from build123d import *

# Parameters (mm, degrees)
SKETCH1_R           = 3.175
BOSS_EXTRUDE1_DEPTH = 25.4
SKETCH2_W           = 6.268193042
SKETCH2_H           = 1.016
BOSS_EXTRUDE2_DEPTH = 6.35
SKETCH3_R           = 1.27
CUT_EXTRUDE1_DEPTH  = 33.120205697
FILLET1_R           = 0.508


with BuildPart() as part:
    # Sketch1 → Boss-Extrude1 (new body)
    with BuildSketch(Plane(origin=(0, 0, 0), x_dir=(0, 0, -1), z_dir=(1, 0, 0))):
        Circle(SKETCH1_R)
    extrude(amount=BOSS_EXTRUDE1_DEPTH)

    # Sketch2 → Boss-Extrude2 (add)
    with BuildSketch(Plane(origin=(25.4, 0, 0), x_dir=(0, 0, -1), z_dir=(1, 0, 0))):
        Rectangle(SKETCH2_W, SKETCH2_H)
    extrude(amount=BOSS_EXTRUDE2_DEPTH)

    # Sketch3 → Cut-Extrude1 (cut, through all)
    with BuildSketch(Plane(origin=(0, 0.508, 0), x_dir=(1, 0, 0), z_dir=(0, 1, 0))):
        with Locations(Location((28.575, 0, 0), (0, 0, 270))):
            Circle(SKETCH3_R)
    extrude(amount=-CUT_EXTRUDE1_DEPTH, mode=Mode.SUBTRACT)

    # Fillet1
    # the kernel refuses this fillet: 0.508 mm, written as the material it adds along each edge
    with BuildSketch(Plane(origin=(25.4, -0.508, -3.134096521), x_dir=(0, -1, 0), z_dir=(0, 0, 1))) as fillet1_piece_1_section:
        with BuildLine():
            CenterArc((FILLET1_R, FILLET1_R), FILLET1_R, 180, 90)
            Line((0, FILLET1_R), (0, 0))
            Line((0, 0), (FILLET1_R, 0))
        make_face()
    fillet1_piece_1 = extrude(amount=6.268193041, mode=Mode.PRIVATE)
    fillet1_piece_1 = fillet1_piece_1 & Plane(origin=(25.515488837, 0, 0), x_dir=(0, 0, -1), z_dir=(-1, 0, 0)) * Cylinder(3.175, 15, mode=Mode.PRIVATE)
    add(fillet1_piece_1)
    with BuildSketch(Plane(origin=(25.4, 0.508, 3.134096521), x_dir=(0, 1, 0), z_dir=(0, 0, -1))) as fillet1_piece_2_section:
        with BuildLine():
            CenterArc((FILLET1_R, FILLET1_R), FILLET1_R, 180, 90)
            Line((0, FILLET1_R), (0, 0))
            Line((0, 0), (FILLET1_R, 0))
        make_face()
    fillet1_piece_2 = extrude(amount=6.268193041, mode=Mode.PRIVATE)
    fillet1_piece_2 = fillet1_piece_2 & Plane(origin=(25.515488837, 0, 0), x_dir=(0, 0, -1), z_dir=(-1, 0, 0)) * Cylinder(3.175, 15, mode=Mode.PRIVATE)
    add(fillet1_piece_2)


solid = part.part
Can you work these out from the model? Positions are in its coordinate system, mm. A direction names the side the tool comes from. Give positions to 0.01 mm unless a question says otherwise; leave off trailing zeros. Order: outer loops, then holes, each group sorted by start corner. A loop starts at its lowest first (then second) coordinate and runs counter-clockwise, first axis right, second up. Notation, with made-up numbers: M 27,2.5 L 59,2.5 A37 cw 59,41.5 Z; hole C 50,12.5 d11. An arc over 180 degrees is marked long. Use one line per item in the form item = value. Start each with the question number.
Item 1: If we section it at B-B (z = -1.75): Write out the boundary of the cut face in (x, y).
Item 2: For faces 1 (the flat face through (30, 0.508, 0)), 2 (the flat face through (29, 0, 3.134)), 3 (the cylindrical face through (12.77, 3.1, 0.69)), 4 (the flat face through (0, 0, 0)), 5 (the flat face through (25.4, -2, 0)), which set-ups out of +Z, -Z, +X, -X, +Y, -Y let a thin tool reach every point of the face, with its end or its side?
Item 3: If we section it at C-C (x = 23.5): Write out the boundary of the cut face in (y, z) (3 decimals).
Item 4: Will these pins go through, and if not, where does the flat tip stop? pin 1 Ø1.1 at (x, y) = (27, 0) entering from -Z; pin 2 Ø3.5 at (x, z) = (28.575, 0) entering from -Y; pin 3 Ø2.5 at (y, z) = (2, 1) entering from +X.
Item 5: If we section it at A-A (z = 0): Write out the boundary of the cut face in (x, y) (3 decimals), then the cut area to 3 significant figures.
Item 6: If I drill on line 1 along X through (y, z) = (-0.2, 0) (3 decimals); line 2 along Z through (x, y) = (12.5, -1); line 3 along Z through (x, y) = (14.5, -0.5), over which ranges is the centre line in solid material (lowest first)?
Item 7: We'd pull the mould along X, two halves only. Please class faces 6 (the cylindrical face through (27.335, 0.007, -0.275)), 7 (the flat face through (29, 0, -3.134)), 8 (the flat face through (25.4, 2, 0)): +X half, -X half, draft (parallel to the pull), parting line (faces both ways), or undercut.
Outcome:
q1.outline = M 0,-2.65 L 25.4,-2.65 L 25.4,-1.02 A0.51 cw 25.91,-0.51 L 31.75,-0.51 L 31.75,0.51 L 25.91,0.51 A0.51 cw 25.4,1.02 L 25.4,2.65 L 0,2.65 Z
q2.face_1 = +Z, -Z, +X, +Y
q2.face_2 = +Z, +X, +Y, -Y
q2.face_3 = +X, -X
q2.face_4 = +Z, -Z, -X, +Y, -Y
q2.face_5 = +Z, -Z, +X, -Y
q3.outline = C 0,0 d6.35
q4.pin_1 = -3.13
q4.pin_2 = -0.51
q4.pin_3 = 25.48
q5.outline = M 0,-3.175 L 25.4,-3.175 L 25.4,-1.016 A0.508 cw 25.908,-0.508 L 27.305,-0.508 L 27.305,0.508 L 25.908,0.508 A0.508 cw 25.4,1.016 L 25.4,3.175 L 0,3.175 Z; M 29.845,-0.508 L 31.75,-0.508 L 31.75,0.508 L 29.845,0.508 Z
q5.area = 165 mm2
q6.line_1 = 0 to 27.305, 29.845 to 31.75
q6.line_2 = -3.01 to 3.01
q6.line_3 = -3.14 to 3.14
q7.face_6 = undercut
q7.face_7 = draft
q7.face_8 = +X half
